Input: part model. Units: mm. Frame: model coordinates. Coordinates: 2 decimals unless noted, no trailing zeros. Loops run counter-clockwise (first coordinate to the right, second up) from the corner with the lowest first, then second, coordinate; pieces in that order, holes last.
(1) Section A-A, the plane x = 0. Return loops of the section in (y, z).
(2) Section C-C, the plane y = 0.25. Return loops of the section in (x, z).
(3) Mould query, pull axis Y, two halves, no side actions, for faces 1 (the face through (0, -5.436, 0)), 2 (the face through (0, 5.436, 0)), 3 (the face through (-1.214, -0.073, -0.931)). Classes: released by +Y, released by -Y, zero draft, split by the parting line, or undercut.
(4) Section B-B, the plane z = 0. Return loops of the section in (x, y), then the cut area to 3 significant figures.
(5) Contact query for a flat-ended pin moving along its axis: P1, Ø1, axis at y = 2, z = 1, coming from the +X side. Output: stop coordinate, or through.
(6) Line query: L1, parallel to Z at x = 0.05, y = 4.5; L2, parallel to X at y = 5, z = 0.45; L3, parallel to Z at x = 0.7, y = 4.75. Output: solid intervals per line, ascending.
```python
from build123d import *

# Parameters (mm, degrees)
F0_R          = 1.5303057729
F1_DEPTH      = 5.1816
F1_DEPTH_BACK = 5.1816
F2_R          = 1.7379746904
F3_DEPTH      = 0.254


# Not quite as in the source:
# - a pattern or mirror of a feature is missing from the dataset's text; its kind, count and spacing are read off the source's solid


with BuildPart() as f1:
    # F0 (on Front) → F1 (new body, two sides)
    with BuildSketch(Plane.XZ) as f1_sk:
        Circle(F0_R)
    extrude(amount=F1_DEPTH)
    extrude(f1_sk.sketch, amount=-F1_DEPTH_BACK)

    # F2 (on face) → F3 (join)
    with BuildSketch(Plane.XZ.offset(5.1816)):
        Circle(F2_R)
    f3 = extrude(amount=F3_DEPTH)

    # F3_copies: F3 across plane
    add(f3.mirror(Plane.ZX))


solid = f1.part
```
Report:
1. outline: (-5.44, -1.74) - (-5.18, -1.74) - (-5.18, -1.53) - (5.18, -1.53) - (5.18, -1.74) - (5.44, -1.74) - (5.44, 1.74) - (5.18, 1.74) - (5.18, 1.53) - (-5.18, 1.53) - (-5.18, 1.74) - (-5.44, 1.74) - close
2. outline: circle Ø3.06 at (0, 0)
3. face 1: released by -Y
3. face 2: released by +Y
3. face 3: undercut
4. outline: (-1.74, -5.44) - (1.74, -5.44) - (1.74, -5.18) - (1.53, -5.18) - (1.53, 5.18) - (1.74, 5.18) - (1.74, 5.44) - (-1.74, 5.44) - (-1.74, 5.18) - (-1.53, 5.18) - (-1.53, -5.18) - (-1.74, -5.18) - close
4. area: 33.5 mm2
5. P1: stops at x = 1.45
6. L1: z = -1.53 to 1.53
6. L2: x = -1.46 to 1.46
6. L3: z = -1.36 to 1.36
